```python
from build123d import *

# Parameters (mm, degrees)
SKETCH1_R           = 1.5
SKETCH1_R_2         = 3
BOSS_EXTRUDE1_DEPTH = 3.175


with BuildPart() as part:
    # Sketch1 → Boss-Extrude1 (new body)
    with BuildSketch(Plane(origin=(0, 0, 0), x_dir=(1, 0, 0), z_dir=(0, 1, 0))):
        Polygon((70, 110.468098835), (450, 110.468098835), (450, 310.468098835), (70, 310.468098835), (70, 325.468098835), (0, 325.468098835), (0, 95.468098835), (70, 95.468098835), align=None)
        with Locations(Location((55, 315.468098835, 0), (0, 0, 270))):
            Circle(SKETCH1_R, mode=Mode.SUBTRACT)
        with Locations(Location((15, 315.468098835, 0), (0, 0, 270))):
            Circle(SKETCH1_R, mode=Mode.SUBTRACT)
        with Locations(Location((55, 105.468098835, 0), (0, 0, 270))):
            Circle(SKETCH1_R, mode=Mode.SUBTRACT)
        with Locations(Location((15, 105.468098835, 0), (0, 0, 270))):
            Circle(SKETCH1_R, mode=Mode.SUBTRACT)
        with Locations(Location((410, 225.468098835, 0), (0, 0, 270))):
            Circle(SKETCH1_R, mode=Mode.SUBTRACT)
        with Locations(Location((410, 195.468098835, 0), (0, 0, 270))):
            Circle(SKETCH1_R, mode=Mode.SUBTRACT)
        with Locations(Location((10, 260.468098835, 0), (0, 0, 270))):
            Circle(SKETCH1_R_2, mode=Mode.SUBTRACT)
        with Locations(Location((440, 300.468098835, 0), (0, 0, 270))):
            Circle(SKETCH1_R_2, mode=Mode.SUBTRACT)
        with Locations(Location((140, 300.468098835, 0), (0, 0, 270))):
            Circle(SKETCH1_R_2, mode=Mode.SUBTRACT)
        with Locations(Location((290, 300.468098835, 0), (0, 0, 270))):
            Circle(SKETCH1_R_2, mode=Mode.SUBTRACT)
        with Locations(Location((440, 120.468098835, 0), (0, 0, 90))):
            Circle(SKETCH1_R_2, mode=Mode.SUBTRACT)
        with Locations(Location((290, 120.468098835, 0), (0, 0, 90))):
            Circle(SKETCH1_R_2, mode=Mode.SUBTRACT)
        with Locations(Location((140, 120.468098835, 0), (0, 0, 90))):
            Circle(SKETCH1_R_2, mode=Mode.SUBTRACT)
        with Locations(Location((10, 120.468098835, 0), (0, 0, 90))):
            Circle(SKETCH1_R_2, mode=Mode.SUBTRACT)
        with Locations(Location((10, 160.468098835, 0), (0, 0, 90))):
            Circle(SKETCH1_R_2, mode=Mode.SUBTRACT)
    extrude(amount=BOSS_EXTRUDE1_DEPTH)


solid = part.part
```
Verification items for the finished model (mm, model axes). Coordinates: 2 decimals unless noted, no trailing zeros. Write each loop counter-clockwise with the first axis right and the second up, starting at its lowest first coordinate (ties: lowest second). Pieces come first, ordered by that corner, then holes. Notation, with made-up numbers: (62, -20) - (110, -20) arc R29 ccw to (110, 2) - close; hole circle Ø10 at (30.25, 26). An arc over 180 degrees is marked (long way). Write item = value, one per line.
Q1. Cross-section at B-B (x = 355). Enter the section's corners in (y, z) (3 decimals), plus the area to 3 significant figures.
Answer:
outline = (0, -310.468) - (3.175, -310.468) - (3.175, -110.468) - (0, -110.468) - close
area = 635 mm²
Q2. Cross-section at A-A (y = 0.8). Give the number of separate pieces and of enclosed holes in the cut face, plus the area to 3 significant figures.
Answer:
separate_pieces = 1
enclosed_holes = 15
area = 91,800 mm²
Q3. Go/stop test with a flat-tipped pin: pin 1 Ø1.6 at (x, y) = (276, 1.5) entering from +Z. Record where the tip stops, or that it passes through.
Answer:
pin_1 = -110.47
Q4. Material ranges on L1, parallel to Z at x = 410, y = 2.25; L2, parallel to X at y = 2.2, z = -300; L3, parallel to X at y = 1, z = -225, recorded low to high. Write a range as from..to.
Answer:
L1 = -310.47..-226.97, -223.97..-196.97, -193.97..-110.47
L2 = 0..137.04, 142.96..287.04, 292.96..437.04, 442.96..450
L3 = 0..408.57, 411.43..450
